Design review of the part built by this model. Coordinates are the model's own, in mm. Coordinates: 2 decimals unless noted, no trailing zeros. One line per item, written item: value.
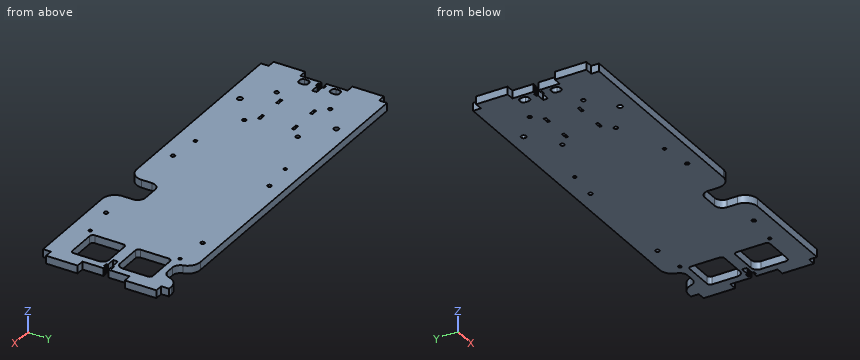
from build123d import *

# Parameters (mm, degrees)
ESQUISSE1_R        = 1
ESQUISSE1_R_2      = 1.25
ESQUISSE1_R_3      = 1.6
ESQUISSE1_W        = 4
ESQUISSE1_H        = 1.5
BOSS_EXTRU_1_DEPTH = 5
SKETCH1_R          = 1.25
SKETCH1_W          = 15
SKETCH1_H          = 10
SKETCH1_W_2        = 5
SKETCH1_H_2        = 6
SKETCH1_W_3        = 20
SKETCH1_H_3        = 20
SKETCH1_W_4        = 22
SKETCH1_H_4        = 22
CUT_EXTRUDE1_DEPTH = 10
FILLET2_R          = 5
FILLET3_R          = 2
CONG_1_R           = 8
CONG_2_R           = 2
CONG_3_R           = 4


with BuildPart() as part:
    # Esquisse1 → Boss.-Extru.1 (new body)
    with BuildSketch(Plane.XY):
        Polygon((0, 35), (0, 15), (5, 15), (5, 1.5), (7, 1.5), (7, 2.6), (9.3, 2.6), (9.3, 1.5), (15, 1.5), (15, -1.5), (9.3, -1.5), (9.3, -2.6), (7, -2.6), (7, -1.5), (5, -1.5), (5, -15), (0, -15), (0, -35), (5, -35), (5, -40), (233, -40), (233, -35), (238, -35), (238, -15), (233, -15), (233, -1.5), (231, -1.5), (231, -2.6), (228.7, -2.6), (228.7, -1.5), (223, -1.5), (223, 1.5), (228.7, 1.5), (228.7, 2.6), (231, 2.6), (231, 1.5), (233, 1.5), (233, 15), (238, 15), (238, 35), (233, 35), (233, 40), (5, 40), (5, 35), align=None)
        with Locations((203, -28.177197641)):
            Circle(ESQUISSE1_R, mode=Mode.SUBTRACT)
        with Locations((203, 28.822802359)):
            Circle(ESQUISSE1_R, mode=Mode.SUBTRACT)
        with Locations((93, -28.177197641)):
            Circle(ESQUISSE1_R, mode=Mode.SUBTRACT)
        with Locations((93, 28.822802359)):
            Circle(ESQUISSE1_R, mode=Mode.SUBTRACT)
        with Locations((112.5, -30.615)):
            Circle(ESQUISSE1_R_2, mode=Mode.SUBTRACT)
        with Locations(Location((42.5, -30.615, 0), (0, 0, 180))):
            Circle(ESQUISSE1_R_3, mode=Mode.SUBTRACT)
        with Locations((182.5, -30.615)):
            Circle(ESQUISSE1_R_2, mode=Mode.SUBTRACT)
        with Locations((42.5, 30.615)):
            Circle(ESQUISSE1_R_3, mode=Mode.SUBTRACT)
        with Locations(Location((182.5, 30.615, 0), (0, 0, 180))):
            Circle(ESQUISSE1_R_2, mode=Mode.SUBTRACT)
        with Locations(Location((112.5, 30.615, 0), (0, 0, 180))):
            Circle(ESQUISSE1_R_2, mode=Mode.SUBTRACT)
        with Locations((34, -10.75)):
            Rectangle(ESQUISSE1_W, ESQUISSE1_H, mode=Mode.SUBTRACT)
        with Locations((34, 10.75)):
            Rectangle(ESQUISSE1_W, ESQUISSE1_H, mode=Mode.SUBTRACT)
        with Locations((53, 10.75)):
            Rectangle(ESQUISSE1_W, ESQUISSE1_H, mode=Mode.SUBTRACT)
        with Locations((53, -10.75)):
            Rectangle(ESQUISSE1_W, ESQUISSE1_H, mode=Mode.SUBTRACT)
    extrude(amount=BOSS_EXTRU_1_DEPTH)

    # Sketch1 → Cut-Extrude1 (cut)
    with BuildSketch(Plane(origin=(0, 0, 0), x_dir=(-1, 0, 0), z_dir=(0, 0, -1))):
        with Locations((-60.5, 17)):
            Circle(SKETCH1_R)
        with Locations((-60.5, -17)):
            Circle(SKETCH1_R)
        with Locations((-26.5, 17)):
            Circle(SKETCH1_R)
        with Locations((-26.5, -17)):
            Circle(SKETCH1_R)
        with Locations((-215.5, 35)):
            Rectangle(SKETCH1_W, SKETCH1_H)
        with Locations((-9.5, 10)):
            Rectangle(SKETCH1_W_2, SKETCH1_H_2)
        with Locations((-153, -30.429903646)):
            Rectangle(SKETCH1_W_3, SKETCH1_H_3)
        with Locations((-9.5, -10)):
            Rectangle(SKETCH1_W_2, SKETCH1_H_2)
        with Locations((-217, 14.5)):
            Rectangle(SKETCH1_W_4, SKETCH1_H_4)
        with Locations((-217, -14.5)):
            Rectangle(SKETCH1_W_4, SKETCH1_H_4)
    extrude(amount=-CUT_EXTRUDE1_DEPTH, mode=Mode.SUBTRACT)

    # Fillet2
    fillet2_edges = [part.edges().sort_by_distance(p)[0] for p in [
        (208, 30, 2.5),
        (223, 30, 2.5),
        (163, -20.429903646, 2.5),
        (143, -20.429903646, 2.5),
    ]]
    fillet(fillet2_edges, radius=FILLET2_R)

    # Fillet3
    fillet3_edges = [part.edges().sort_by_distance(p)[0] for p in [
        (228, -25.5, 2.5),
        (206, -3.5, 2.5),
        (206, -25.5, 2.5),
        (228, 25.5, 2.5),
        (206, 25.5, 2.5),
        (206, 3.5, 2.5),
    ]]
    fillet(fillet3_edges, radius=FILLET3_R)

    # Congé1
    cong_1_edges = [part.edges().sort_by_distance(p)[0] for p in [
        (223, 40, 2.5),
        (208, 40, 2.5),
        (163, -40, 2.5),
        (143, -40, 2.5),
    ]]
    fillet(cong_1_edges, radius=CONG_1_R)

    # Congé2
    cong_2_edges = [part.edges().sort_by_distance(p)[0] for p in [
        (12, 7, 2.5),
        (12, 13, 2.5),
        (7, 13, 2.5),
        (7, 7, 2.5),
        (7, -13, 2.5),
        (12, -13, 2.5),
        (12, -7, 2.5),
        (7, -7, 2.5),
    ]]
    fillet(cong_2_edges, radius=CONG_2_R)

    # Congé3
    cong_3_edges = [part.edges().sort_by_distance(p)[0] for p in [
        (228, -3.5, 2.5),
        (228, 3.5, 2.5),
    ]]
    fillet(cong_3_edges, radius=CONG_3_R)


solid = part.part
1. Wall thickness on line 1 along Y through (x, z) = (182.5, 2.95) (3 decimals); line 2 along Y through (x, z) = (60.5, 3.75); line 3 along X through (y, z) = (-9, 3.2): over which ranges is each line inside the solid? List them lowest first.
Answer block:
line 1: y = -40 to -31.865, -29.365 to 29.365, 31.865 to 40
line 2: y = -40 to -18.25, -15.75 to 15.75, 18.25 to 40
line 3: x = 5 to 7, 12 to 206, 228 to 233
2. Consider section A-A, the plane z = 1.9. Give the number of separate pieces and of enclosed holes in the cut face, then the cut area to 3 significant figures.
Answer block:
separate pieces: 1
enclosed holes: 22
area: 16,900 mm^2
3. Insertion check: pin 1 Ø1.5 at (x, z) = (2, 2.5) entering from -Y; pin 2 Ø1.2 at (y, z) = (-10.5, 2) entering from +X; pin 3 Ø0.8 at (y, z) = (-11, 2) entering from -X. Each pin has a flat end and moves straight along its axis. Give the tip position at first contact, or say it passes through.
Answer block:
pin 1: stops at y = -35
pin 2: stops at x = 233
pin 3: stops at x = 5
